CAD build for the part. Positions are in the model's coordinates, mm. A direction names the side the tool comes from. Give positions to 0.01 mm unless a question says otherwise; leave off trailing zeros. Loops run counter-clockwise (first coordinate to the right, second up) from the corner with the lowest first, then second, coordinate; pieces in that order, holes last.
```python
from build123d import *

# Parameters (mm, degrees)
SKETCH1_R           = 2.54
BOSS_EXTRUDE1_DEPTH = 15.24
SKETCH2_R           = 1.375
CUT_EXTRUDE1_DEPTH  = 12.7
SKETCH4_R           = 1.5875
SKETCH4_R_2         = 1.3335
EXTRUDE_THIN1_DEPTH = 1.27


with BuildPart() as part:
    # Sketch1 → Boss-Extrude1 (new body)
    with BuildSketch(Plane(origin=(0, 0, 0), x_dir=(1, 0, 0), z_dir=(0, 1, 0))):
        with Locations(Location((0, 0, 0), (0, 0, 90))):
            Circle(SKETCH1_R)
    extrude(amount=BOSS_EXTRUDE1_DEPTH)

    # Sketch2 → Cut-Extrude1 (cut)
    with BuildSketch(Plane(origin=(0, 15.24, 0), x_dir=(1, 0, 0), z_dir=(0, 1, 0))):
        with Locations(Location((0, 0, 0), (0, 0, 270))):
            Circle(SKETCH2_R)
    extrude(amount=-CUT_EXTRUDE1_DEPTH, mode=Mode.SUBTRACT)

    # Sketch4 → Extrude-Thin1 (add)
    with BuildSketch(Plane.XZ):
        Circle(SKETCH4_R)
        Circle(SKETCH4_R_2, mode=Mode.SUBTRACT)
    extrude(amount=EXTRUDE_THIN1_DEPTH)


solid = part.part
```
1. Probe line 1 along Y through (x, z) = (0.85, 1.8); line 2 along Z through (x, y) = (-0.25, 6.5); line 3 along X through (y, z) = (4.5, -0.45). List the from-to ranges inside material, lowest first.
Responses:
line 1: y = 0 to 15.24
line 2: z = -2.53 to -1.35, 1.35 to 2.53
line 3: x = -2.5 to -1.3, 1.3 to 2.5
2. Saw through at D-D, the plane x = 2.05. List the corners of the cut face in (y, z), and give its area (3 significant figures).
Responses:
outline: (0, -1.5) - (15.24, -1.5) - (15.24, 1.5) - (0, 1.5) - close
area: 45.7 mm2
3. Saw through at C-C, the plane y = 6.5. List the corners of the cut face in (x, z) (3 decimals), and give its area (3 significant figures).
Responses:
outline: circle Ø5.08 at (0, 0); hole circle Ø2.75 at (0, 0)
area: 14.3 mm2
4. Pull direction X, two halves, no side cores. Call faces 1 (the face through (0.62, -0.63, -1.18)), 2 (the face through (0, 0, 0)), 3 (the face through (-2.52, 7.51, 0.33)), 4 (the face through (1.1, 15.24, -1.1)): released by +X, released by -X, zero draft, split by the parting line, or undercut.
Responses:
face 1: undercut
face 2: undercut
face 3: split by the parting line
face 4: zero draft
5. Tool access for faces 5 (the face through (0, 2.54, 0)), 6 (the face through (2, 0, 0)): list every direction of +Z, -Z, +X, -X, +Y, -Y with a clear straight run to the whole face (end or side of a thin tool).
Responses:
face 5: +Y
face 6: -Y
6. Drop flat-ended pins along their axis: pin 1 (2 mm diameter, centred on x = -1.5, y = 12, fed in from +Z); pin 2 (2 mm diameter, centred on y = 3.5, z = 0.5, fed in from -X); pin 3 (1.6 mm diameter, centred on x = 0, z = 0, fed in from -Y). Give the stop position or say it passes through.
Responses:
pin 1: stops at z = 2.49
pin 2: stops at x = -2.54
pin 3: stops at y = 0
